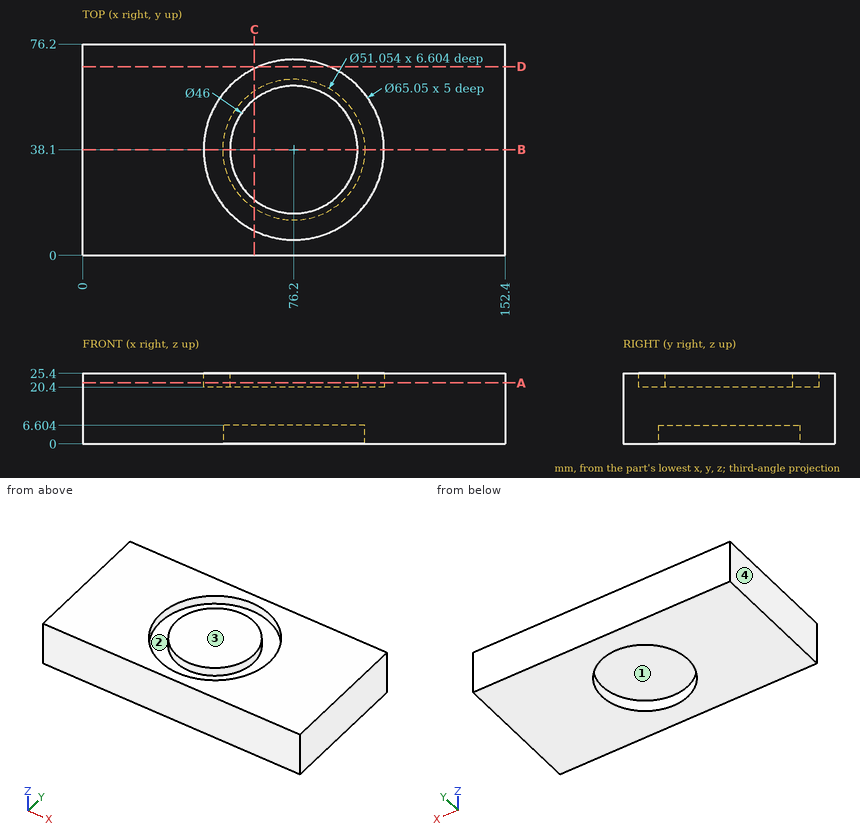
Input: dimensioned drawing with shaded views. Units: mm. Origin: part minimum x, y, z. Give positions to 0.01 mm unless a question says otherwise; leave off trailing zeros. Write each loop counter-clockwise with the first axis right and the second up, starting at its lowest first coordinate (ties: lowest second). Pieces come first, ordered by that corner, then holes.
Q1. Pull-direction query (X, two-part tool) for the marked faces 1, 2, 3 and 4; classes: pulls with the +X half, pulls with the -X half, needs draft (parallel to the pull), parting line crosses it, or undercut.
Q2. Material intervals for probe 1 along X at (y, z) = (38.1, 4.5); probe 2 along Y at (x, z) = (76.2, 22.55) (3 decimals); probe 3 along Y at (x, z) = (57.5, 23.75), sorted ascending.
Q3. Section D-D, the plane y = 68. Output: boundary loops of the cut face in (x, z).
Q4. Section B-B, the plane y = 38.1. Output: boundary loops of the cut face in (x, z) (3 decimals), plus the area to 3 significant figures.
Q5. Section A-A, the plane z = 22. Output: boundary loops of the cut face in (x, y) (3 decimals), plus the area to 3 significant figures.
Q6. Section C-C, the plane x = 62. Output: boundary loops of the cut face in (y, z), plus the area to 3 significant figures.
Filled in:
1. face 1: undercut
1. face 2: undercut
1. face 3: needs draft
1. face 4: pulls with the -X half
2. probe 1: x = 0 to 50.67, 101.73 to 152.4
2. probe 2: y = 0 to 5.575, 15.1 to 61.1, 70.625 to 76.2
2. probe 3: y = 0 to 11.49, 24.71 to 51.49, 64.71 to 76.2
3. outline: (0, 0) - (152.4, 0) - (152.4, 25.4) - (89, 25.4) - (89, 20.4) - (63.4, 20.4) - (63.4, 25.4) - (0, 25.4) - close
4. outline: (0, 0) - (50.673, 0) - (50.673, 6.604) - (101.727, 6.604) - (101.727, 0) - (152.4, 0) - (152.4, 25.4) - (108.725, 25.4) - (108.725, 20.4) - (99.2, 20.4) - (99.2, 25.4) - (53.2, 25.4) - (53.2, 20.4) - (43.675, 20.4) - (43.675, 25.4) - (0, 25.4) - close
4. area: 3,440 mm2
5. outline: (0, 0) - (152.4, 0) - (152.4, 76.2) - (0, 76.2) - close; circle Ø46 at (76.2, 38.1); hole circle Ø65.05 at (76.2, 38.1)
5. area: 9,950 mm2
6. outline: (0, 0) - (16.89, 0) - (16.89, 6.6) - (59.31, 6.6) - (59.31, 0) - (76.2, 0) - (76.2, 25.4) - (67.36, 25.4) - (67.36, 20.4) - (56.19, 20.4) - (56.19, 25.4) - (20.01, 25.4) - (20.01, 20.4) - (8.84, 20.4) - (8.84, 25.4) - (0, 25.4) - close
6. area: 1,540 mm2
